Autodesk Inventor part; units mm, degrees
ref_plane "YZ Plane" through (0, 0, 0) normal (1, 0, 0) x (0, 1, 0)
ref_plane "XZ Plane" through (0, 0, 0) normal (0, 1, 0) x (-1, 0, 0)
ref_plane "XY Plane" through (0, 0, 0) normal (0, 0, 1) x (1, 0, 0)
sketch "Sketch1" plane through (0, 0, 0) normal (0, 1, 0) x (-1, 0, 0)
  circle A0 centre (0, 0) radius 2.75
  arc A1 (0, -7.75) -> (-7.75, 0) centre (0, 0) ccw
  line L0 (0, 0) -> (-30, 0)
  line L1 (0, -7.75) -> (-14.1906, -7.75)
  line L2 (-30, 0) -> (-30, -20) construction
  arc A2 (-18.8169, -15) -> (-41.1831, -15) centre (-30, -20) ccw
  line L3 (-30, 0) -> (-30, -15) construction
  line L4 (-41.1831, -15) -> (-49.3649, -15)
  line L5 (-18.8169, -15) -> (-10.6351, -15)
  arc A3 (-10.6351, -15) -> (-14.1906, -7.75) centre (-30, -20) ccw
  arc A4 (-30, 0) -> (-49.3649, -15) centre (-30, -20) ccw
  dimension "d0" = 5.5
  dimension "d1" = 5
  dimension "d2" = 30
  dimension "d3" = 20
  dimension "d4" = 15
extrude "Extrusion1" add sketch "Sketch1" along normal blind 5
sketch "Sketch2" plane through (0, 5, 0) normal (0, 1, 0) x (1, 0, 0)
  arc A0 (18.8169, 15) -> (41.1831, 15) centre (30, 20) ccw
  circle A1 centre (30, 20) radius 12.25
  line L0 (7.75, 0) -> (30, 0)
  circle A2 centre (30, 20) radius 20
  line L1 (49.3649, 15) -> (41.1831, 15)
  line L2 (49.3649, 15) -> (10.6351, 15)
  point P0 (0, 0)
extrude "Extrusion2" add sketch "Sketch2" along normal blind 5 contours A0 L1 A2 L2
sketch "Sketch3" plane through (0, 0, 0) normal (0, -1, 0) x (1, 0, 0)
  circle A0 centre (0, 0) radius 5
  dimension "d9" = 10
extrude "Extrusion3" cut sketch "Sketch3" against normal blind 3
properties part number "CameraMount" material "ABS Plastic"
CAD build for the part. Positions are in the model's coordinates, mm. A direction names the side the tool comes from. Give positions to 0.01 mm unless a question says otherwise; leave off trailing zeros. Loops run counter-clockwise (first coordinate to the right, second up) from the corner with the lowest first, then second, coordinate; pieces in that order, holes last. Notation, with made-up numbers: M 72,64.25 L 126,64.25 A21 cw 126,86.25 Z; hole C -33,82.5 d4. An arc over 180 degrees is marked long. Answer in a Markdown table with one row per item. Add a question column.
Item 1: Band-saw the part on C-C on x = 19.5. Give the cut face in (y, z).
Item 2: Tool access for faces 1 (the face through (15, 5, -15)), 2 (the face through (7, 2, -7.75)), 3 (the face through (-1.08, 1.48, -4.88)), 4 (the face through (3, 5, -2)), 5 (the face through (-5.296, 2.465, 5.658)): list every direction of +Z, -Z, +X, -X, +Y, -Y with a clear straight run to the whole face (end or side of a thin tool).
Item 3: Band-saw the part on D-D on y = 9.25. Give the cut face in (x, z).
Item 4: Mould opens along X. For faces 6 (the face through (30, 7, 0)), 7 (the face through (19, 2, 0)), 8 (the face through (2.2, 3, -2.2)), 9 (the face through (42, 2, -4)) say: +X half, -X half, draft (parallel to the pull), parting line (faces both ways), or undercut.
Item 5: Band-saw the part on B-B on z = -2. Give the cut face in (x, y), then the cut area to 3 significant figures.
Item 6: Probe probe 1 along Z at (x, y) = (0, 4.2); probe 2 along Y at (x, z) = (-3.5, -2.5); probe 3 along Z at (x, y) = (0, 1.6). List the from-to ranges inside material, lowest first.
Item 7: Drop flat-ended pins along their axis: P1, Ø6, axis at x = 33, y = 4, coming from the -Z side; P2, Ø6, axis at y = 3, z = -8.5, coming from the -X side; P3, Ø2, axis at y = 4.5, z = 2.5, coming from the -X side. Give the stop position or say it passes through.
Item 8: Band-saw the part on A-A on y = 1.25. Give the cut face in (x, z), then the cut area to 3 significant figures.
Reply:
| question | item | result |
|---|---|---|
| 1 | outline | M 0,-13.69 L 10,-13.69 L 10,-2.98 L 5,-2.98 L 5,0 L 0,0 Z |
| 2 | face 1 | -Z, +X, -X, +Y, -Y |
| 2 | face 2 | -X, +Y, -Y |
| 2 | face 3 | -Y |
| 2 | face 4 | +Z, -X, +Y |
| 2 | face 5 | +Y, -Y |
| 3 | outline | M 10.64,-15 L 18.82,-15 A12.25 cw 41.18,-15 L 49.36,-15 A20 ccw Z |
| 4 | face 6 | parting line |
| 4 | face 7 | draft |
| 4 | face 8 | undercut |
| 4 | face 9 | +X half |
| 5 | outline | M -7.49,0 L -4.58,0 L -4.58,3 L -1.89,3 L -1.89,5 L -7.49,5 Z; M 1.89,3 L 4.58,3 L 4.58,0 L 38.72,0 L 38.72,10 L 21.28,10 L 21.28,5 L 1.89,5 Z |
| 5 | area | 283 mm^2 |
| 6 | probe 1 | z = -7.75 to -2.75, 2.75 to 7.75 |
| 6 | probe 2 | y = 3 to 5 |
| 6 | probe 3 | z = -7.75 to -5, 5 to 7.75 |
| 7 | P1 | stops at z = -9.32 |
| 7 | P2 | stops at x = -5.46 |
| 7 | P3 | stops at x = -7.6 |
| 8 | outline | M 0,-7.75 L 14.19,-7.75 A20 ccw 10.64,-15 L 18.82,-15 A12.25 cw 41.18,-15 L 49.36,-15 A20 ccw 30,0 L 7.75,0 A7.75 ccw long Z; hole C 0,0 d10 |
| 8 | area | 524 mm^2 |
